from build123d import *

# Parameters (mm, degrees)
SKETCH_1_W          = 28
SKETCH_1_H          = 28
EXTRUDE_1_DEPTH     = 20
CUT_EXTRUDE_1_DEPTH = 20
SKETCH_3_W          = 24
SKETCH_3_H          = 14.4
CUT_EXTRUDE_2_DEPTH = 24
SKETCH_4_R          = 2.25
CUT_EXTRUDE_3_DEPTH = 10
SKETCH_5_R          = 2.25
CUT_EXTRUDE_4_DEPTH = 10


with BuildPart() as part:
    # 草图1 → 凸台-拉伸1 (new body)
    with BuildSketch(Plane.XY):
        with Locations((14, 14)):
            Rectangle(SKETCH_1_W, SKETCH_1_H)
    extrude(amount=EXTRUDE_1_DEPTH)

    # 草图2 → 切除-拉伸1 (cut)
    with BuildSketch(Plane.XY.offset(20)):
        Polygon((21.5, 28), (21.5, 24), (4, 6.5), (0, 6.5), (0, 28), align=None)
    extrude(amount=-CUT_EXTRUDE_1_DEPTH, mode=Mode.SUBTRACT)

    # 草图3 → 切除-拉伸2 (cut)
    with BuildSketch(Plane(origin=(0, 28, 0), x_dir=(1, 0, 0), z_dir=(0, 1, 0))):
        with Locations((12, -10)):
            Rectangle(SKETCH_3_W, SKETCH_3_H)
    extrude(amount=-CUT_EXTRUDE_2_DEPTH, mode=Mode.SUBTRACT)

    # 草图4 → 切除-拉伸3 (cut)
    with BuildSketch(Plane.XZ):
        with Locations(Location((10, 10, 0), (0, 0, 270))):
            Circle(SKETCH_4_R)
    extrude(amount=-CUT_EXTRUDE_3_DEPTH, mode=Mode.SUBTRACT)

    # 草图5 → 切除-拉伸4 (cut)
    with BuildSketch(Plane(origin=(28, 0, 0), x_dir=(0, 0, -1), z_dir=(1, 0, 0))):
        with Locations((-10, 18)):
            Circle(SKETCH_5_R)
    extrude(amount=-CUT_EXTRUDE_4_DEPTH, mode=Mode.SUBTRACT)


solid = part.part
Geometry: final body of the model. Coordinates: model frame, mm. A direction names the side the tool comes from. Round coordinates to 2 decimals unless told otherwise and drop trailing zeros. Loops run counter-clockwise (first coordinate to the right, second up) from the corner with the lowest first, then second, coordinate; pieces in that order, holes last. Notation, with made-up numbers: M 30,44 L 36,44 A12 ccw 36,63 Z; hole C 86,-38.75 d5. An arc over 180 degrees is marked long. Put each result on its own line as item: value. Start each with the question number.
(1) Contact query for flat-ended pins moving along their axis: pin 1 Ø1 at (y, z) = (12.5, 4) entering from -X; pin 2 Ø3.5 at (x, z) = (10, 10) entering from +Y; pin 3 Ø2 at (y, z) = (26.5, 2) entering from -X; pin 4 Ø7 at (x, z) = (6, 12.5) entering from +Y. Output: stop coordinate, or through.
(2) Set-up query: faces 4 (the face through (21.5, 26, 19)), 5 (the face through (28, 14, 10)), 6 (the face through (12, 4, 8)). Return all of +Z, -Z, +X, -X, +Y, -Y with unobstructed straight access to the full face (end or side cutting, diameter ignored); none if empty.
(3) Section query A-A (z = 10). Return loops of the section in (x, y).
(4) Section query D-D (y = 21). Return loops of the section in (x, z), then the cut area to 3 significant figures.
(5) Material intervals for line 1 along X through (y, z) = (1, 10); line 2 along Z through (x, y) = (13.5, 13.75); line 3 along Y through (x, z) = (25.5, 10), sorted ascending. Write a range as [from, to].
(6) Section query C-C (x = 6). Return loops of the section in (y, z).
(7) Draft query along Z for faces 1 (the face through (17, 11, 0)), 2 (the face through (24, 16, 12)), 3 (the face through (12.9, 15.4, 1.4)). Return one class per face: +Z half, -Z half, draft (parallel to the pull), parting line (faces both ways), or undercut.
(8) Section query B-B (y = 18). Return loops of the section in (x, z).
Findings below:
1. pin 1: stops at x = 24
1. pin 2: passes through
1. pin 3: stops at x = 21.5
1. pin 4: stops at y = 4
2. face 4: +Z, -Z, -X, +Y
2. face 5: +Z, -Z, +X, +Y, -Y
2. face 6: -X, +Y
3. outline: M 0,0 L 7.75,0 L 7.75,4 L 0,4 Z; M 12.25,0 L 28,0 L 28,15.75 L 24,15.75 L 24,4 L 12.25,4 Z; M 24,20.25 L 28,20.25 L 28,28 L 24,28 Z
4. outline: M 18.5,0 L 28,0 L 28,20 L 18.5,20 L 18.5,17.2 L 24,17.2 L 24,2.8 L 18.5,2.8 Z
4. area: 111 mm2
5. line 1: x = [0, 7.75], [12.25, 28]
5. line 2: z = [0, 2.8], [17.2, 20]
5. line 3: y = [0, 15.75], [20.25, 28]
6. outline: M 0,0 L 8.5,0 L 8.5,2.8 L 4,2.8 L 4,17.2 L 8.5,17.2 L 8.5,20 L 0,20 Z
7. face 1: -Z half
7. face 2: undercut
7. face 3: draft
8. outline: M 15.5,0 L 28,0 L 28,7.75 L 24,7.75 L 24,2.8 L 15.5,2.8 Z; M 15.5,17.2 L 24,17.2 L 24,12.25 L 28,12.25 L 28,20 L 15.5,20 Z
